Work out the finished part from the listing and answer in its coordinate system (mm). A direction names the side the tool comes from. Coordinates: 2 decimals unless noted, no trailing zeros. Loops run counter-clockwise (first coordinate to the right, second up) from the corner with the lowest first, then second, coordinate; pieces in that order, holes last. Notation, with made-up numbers: (60, 85) -> (106, 85) arc R27 ccw to (106, 114) -> close; hole circle Ø2 at (1, 31). An arc over 180 degrees is marked (long way). One line per question, with ' | ' between items.
```python
from build123d import *

# Parameters (mm, degrees)
SKETCH1_W           = 71
SKETCH1_H           = 30
BOSS_EXTRUDE1_DEPTH = 3
SKETCH2_R           = 1.25
CUT_EXTRUDE1_DEPTH  = 5
FILLET1_R           = 8
SKETCH3_R           = 7
SKETCH3_R_2         = 1.25
BOSS_EXTRUDE2_DEPTH = 2.5
SKETCH4_R           = 1
CUT_EXTRUDE2_DEPTH  = 10
CIRPATTERN1_COUNT   = 6


with BuildPart() as part:
    # Sketch1 → Boss-Extrude1 (new body)
    with BuildSketch(Plane(origin=(0, 0, 0), x_dir=(0, 0, -1), z_dir=(1, 0, 0))):
        Rectangle(SKETCH1_W, SKETCH1_H)
    extrude(amount=BOSS_EXTRUDE1_DEPTH)

    # Sketch2 → Cut-Extrude1 (cut)
    with BuildSketch(Plane(origin=(3, 0, 0), x_dir=(0, 0, -1), z_dir=(1, 0, 0))):
        with Locations((-27.31, 7)):
            Circle(SKETCH2_R)
        with Locations((0, -4.5)):
            Circle(SKETCH2_R)
        with Locations((-16, -4.5)):
            Circle(SKETCH2_R)
    cut_extrude1 = extrude(amount=-CUT_EXTRUDE1_DEPTH, mode=Mode.SUBTRACT)

    # Mirror1: Cut-Extrude1 across plane
    add(cut_extrude1.mirror(Plane.XY), mode=Mode.SUBTRACT)

    # Fillet1
    fillet1_edges = [part.edges().sort_by_distance(p)[0] for p in [
        (1.5, 15, 35.5),
        (1.5, 15, -35.5),
    ]]
    fillet(fillet1_edges, radius=FILLET1_R)

    # Sketch3 → Boss-Extrude2 (add)
    with BuildSketch(Plane(origin=(0, 0, 0), x_dir=(0, 0, -1), z_dir=(1, 0, 0))):
        with Locations((-27.31, 7)):
            Circle(SKETCH3_R)
        with Locations((-27.31, 7)):
            Circle(SKETCH3_R_2, mode=Mode.SUBTRACT)
    extrude(amount=-BOSS_EXTRUDE2_DEPTH)

    # Sketch4 → Cut-Extrude2 (cut)
    with BuildSketch(Plane.ZY.offset(2.5)):
        with Locations((27.31, 12)):
            Circle(SKETCH4_R)
    cut_extrude2 = extrude(amount=-CUT_EXTRUDE2_DEPTH, mode=Mode.SUBTRACT)

    # CirPattern1: Cut-Extrude2 ×6 about axis
    cirpattern1_axis = Axis((0, 7, 27.31), (1, 0, 0))
    for i in range(1, CIRPATTERN1_COUNT):
        add(cut_extrude2.rotate(cirpattern1_axis, i * 360 / CIRPATTERN1_COUNT), mode=Mode.SUBTRACT)


solid = part.part
```
1) Find section B-B (y = -4.5). Write down the section's boundary in (x, z).
Check values:
outline: (0, -35.5) -> (3, -35.5) -> (3, -17.25) -> (0, -17.25) -> close; (0, -14.75) -> (3, -14.75) -> (3, -1.25) -> (0, -1.25) -> close; (0, 1.25) -> (3, 1.25) -> (3, 14.75) -> (0, 14.75) -> close; (0, 17.25) -> (3, 17.25) -> (3, 35.5) -> (0, 35.5) -> close
2) Flat-ended cylindrical pins translate along their axes: pin 1 (2 mm diameter, centred on y = 7, z = 27.31, fed in from +X); pin 2 (1 mm diameter, centred on x = -1.5, y = 6.5, fed in from -Z); pin 3 (15 mm diameter, centred on y = 1.5, z = -11.5, fed in from -X). Find the tip coordinate at first contact, or state that the pin passes through.
Check values:
pin 1: passes through | pin 2: stops at z = 20.31 | pin 3: stops at x = 0
3) Find the intervals of material crossed by line 1 along Z through (x, y) = (-0.85, 9); line 2 along Z through (x, y) = (1.7, 4.75); line 3 along X through (y, z) = (1.5, -28), in increasing order.
Check values:
line 1: z = 20.6 to 22.11, 23.85 to 30.77, 32.51 to 34.02 | line 2: z = -35.5 to 22.01, 23.95 to 30.67, 32.61 to 35.5 | line 3: x = 0 to 3
4) Find section C-C (x = 2.1). State how many separate pieces and enclosed holes the cut face has, plus the area to 3 significant figures.
Check values:
separate pieces: 1 | enclosed holes: 11 | area: 2,060 mm^2
5) The mould has two halves that part along Y. Classify faces 1 (the face through (1.52, -5.26, 16.99)), 2 (the face through (1.521, 12.594, -33.219)), 3 (the face through (1, -4, 35.5)): released by +Y, released by -Y, zero draft, split by the parting line, or undercut.
Check values:
face 1: undercut | face 2: released by +Y | face 3: zero draft
6) Find section A-A (z = 16). Write down the section's boundary in (x, y), plus the area to 3 significant figures.
Check values:
outline: (0, -15) -> (3, -15) -> (3, -5.75) -> (0, -5.75) -> close; (0, -3.25) -> (3, -3.25) -> (3, 15) -> (0, 15) -> close | area: 82.5 mm^2
7) Find section D-D (y = 2). Write down the section's boundary in (x, z).
Check values:
outline: (-2.5, 22.41) -> (0, 22.41) -> (0, -35.5) -> (3, -35.5) -> (3, 26.31) -> (-2.5, 26.31) -> close; (-2.5, 28.31) -> (3, 28.31) -> (3, 35.5) -> (0, 35.5) -> (0, 32.21) -> (-2.5, 32.21) -> close
8) For faces 4 (the face through (-1.232, 0.166, 28.827)), 5 (the face through (0.288, 6.521, 26.155)), determine the directions among +Z, -Z, +X, -X, +Y, -Y from which every point of the face is accessible in a straight line to the end or side of a thin tool.
Check values:
face 4: -X | face 5: +X, -X
